```python
from build123d import *

# Parameters (mm, degrees)
SKETCH1_W                                 = 9.525
SKETCH1_H                                 = 19.05
BOSS_EXTRUDE1_DEPTH                       = 2
CSK_FOR_0_FLAT_HEAD_MACHINE_SCREW_2_COUNT = 2
CSK_FOR_0_FLAT_HEAD_MACHINE_SCREW_2_PITCH = 4.7625
F_1_8_0_125_DIAMETER_HOLE1_D              = 3.175
F_1_8_0_125_DIAMETER_HOLE1_DEPTH          = 4.064
F_1_8_0_125_DIAMETER_HOLE1_TIP            = 0.953866233


with BuildPart() as part:
    # Sketch1 → Boss-Extrude1 (new body)
    with BuildSketch(Plane.XY):
        Rectangle(SKETCH1_W, SKETCH1_H)
    extrude(amount=BOSS_EXTRUDE1_DEPTH)

    # Sketch2 → CSK for #0 Flat Head Machine Screw (100)1 (revolve, cut)
    with BuildSketch(Plane(origin=(-2.38125, -7.14375, 2), x_dir=(0, -1, 0), z_dir=(1, 0, 0))):
        Polygon((0, 0), (0, 2), (0.889, 2), (0.889, 1.008067835), (1.7653, 0), align=None)
    csk_for_0_flat_head_machine_screw_100 = revolve(axis=Axis((-2.38125, -7.14375, 8.35), (0, 0, -1)), mode=Mode.SUBTRACT)

    # CSK for _0 Flat Head Machine Screw _ 2: CSK for #0 Flat Head Machine Screw (100)1 ×2
    with Locations(*[(i * CSK_FOR_0_FLAT_HEAD_MACHINE_SCREW_2_PITCH, 0, 0) for i in range(1, CSK_FOR_0_FLAT_HEAD_MACHINE_SCREW_2_COUNT)]):
        add(csk_for_0_flat_head_machine_screw_100, mode=Mode.SUBTRACT)

    # 1/8 (0.125) Diameter Hole1
    with Locations(Plane.XY.offset(2)):
        with Locations((0, 6.35), (0, -0.2032)):
            Hole(F_1_8_0_125_DIAMETER_HOLE1_D / 2, depth=F_1_8_0_125_DIAMETER_HOLE1_DEPTH)
            with Locations((0, 0, -(F_1_8_0_125_DIAMETER_HOLE1_DEPTH + F_1_8_0_125_DIAMETER_HOLE1_TIP / 2))):  # 118° drill point
                Cone(0, F_1_8_0_125_DIAMETER_HOLE1_D / 2, F_1_8_0_125_DIAMETER_HOLE1_TIP, mode=Mode.SUBTRACT)


solid = part.part
```
The listing builds one solid part. Answer for the finished solid, in the listing's coordinates (mm). Round coordinates to 2 decimals unless told otherwise and drop trailing zeros. Order: outer loops, then holes, each group sorted by start corner. A loop starts at its lowest first (then second) coordinate and runs counter-clockwise, first axis right, second up. Notation, with made-up numbers: (61, 34.25) -> (113, 34.25) arc R17 cw to (113, 64.25) -> close; hole circle Ø11 at (-16, 87). An arc over 180 degrees is marked (long way). Answer as CSV lines item,"result". Start each with the question number.
(1) The part is cut by section A-A (x = 0). Determine the outline of the cut face in (y, z) (1 decimal).
(2) Find the intervals of material crossed by probe 1 along Y at (x, z) = (0, 0.95) (1 decimal); probe 2 along X at (y, z) = (-6.5, 0.2); probe 3 along Y at (x, z) = (-0.5, 0.45) (1 decimal), in increasing order. Write a range as from..to.
(3) For a pull along Y with two mould halves and no side action, classify faces 1 (the face through (1.26, -1.17, 0.99)), 2 (the face through (0, -9.525, 1)), 3 (the face through (4.762, 0, 1)), 4 (the face through (0, 9.525, 1)) as +Y half, -Y half, draft (parallel to the pull), parting line (faces both ways), or undercut.
(4) The part is cut by section C-C (z = 0.75). Count the separate pieces of the cut face and the enclosed holes in it, then the cut area to 3 significant figures.
(5) The part is cut by section B-B (y = 6.35). Determine the outline of the cut face in (x, z), then the cut area to 3 significant figures.
Evaluation:
1,outline,"(-9.5, 0) -> (-1.8, 0) -> (-1.8, 2) -> (-9.5, 2) -> close; (1.4, 0) -> (4.8, 0) -> (4.8, 2) -> (1.4, 2) -> close; (7.9, 0) -> (9.5, 0) -> (9.5, 2) -> (7.9, 2) -> close"
2,probe 1,"-9.5..-1.8, 1.4..4.8, 7.9..9.5"
2,probe 2,"-4.76..-2.99, -1.77..1.77, 2.99..4.76"
2,probe 3,"-9.5..-1.7, 1.3..4.8, 7.9..9.5"
3,face 1,"undercut"
3,face 2,"-Y half"
3,face 3,"draft"
3,face 4,"+Y half"
4,separate pieces,"1"
4,enclosed holes,"4"
4,area,"161 mm²"
5,outline,"(-4.76, 0) -> (-1.59, 0) -> (-1.59, 2) -> (-4.76, 2) -> close; (1.59, 0) -> (4.76, 0) -> (4.76, 2) -> (1.59, 2) -> close"
5,area,"12.7 mm²"
